Drawing for the job (mm, zero at the part's lowest x, y, z). Give positions to 0.01 mm unless a question says otherwise; leave off trailing zeros. Loops run counter-clockwise (first coordinate to the right, second up) from the corner with the lowest first, then second, coordinate; pieces in that order, holes last.
1) Band-saw the part on C-C on y = 2.45. List the corners of the cut face in (x, z).
2) Two-plate mould, pull along X, no slides. Class the marked faces 1, 2 and 3: +X half, -X half, draft (parallel to the pull), parting line (faces both ways), or undercut.
3) Band-saw the part on B-B on z = 28. List the corners of the cut face in (x, y).
4) Band-saw the part on A-A on x = 28. List the corners of the cut face in (y, z), then the cut area to 3 significant figures.
5) Wall check: line 1 (X direction, y = 3.95, z = 28); line 2 (X direction, y = 1.55, z = 34); line 3 (Z direction, x = 38.5, y = 4.9). Give the ranges that are in metal, low to high.
6) Flat gauge pin, fed straight in: P1, Ø3, axis at y = 4.5, z = 42, coming from the +X side. Where does the tip first touch, or does it go through?
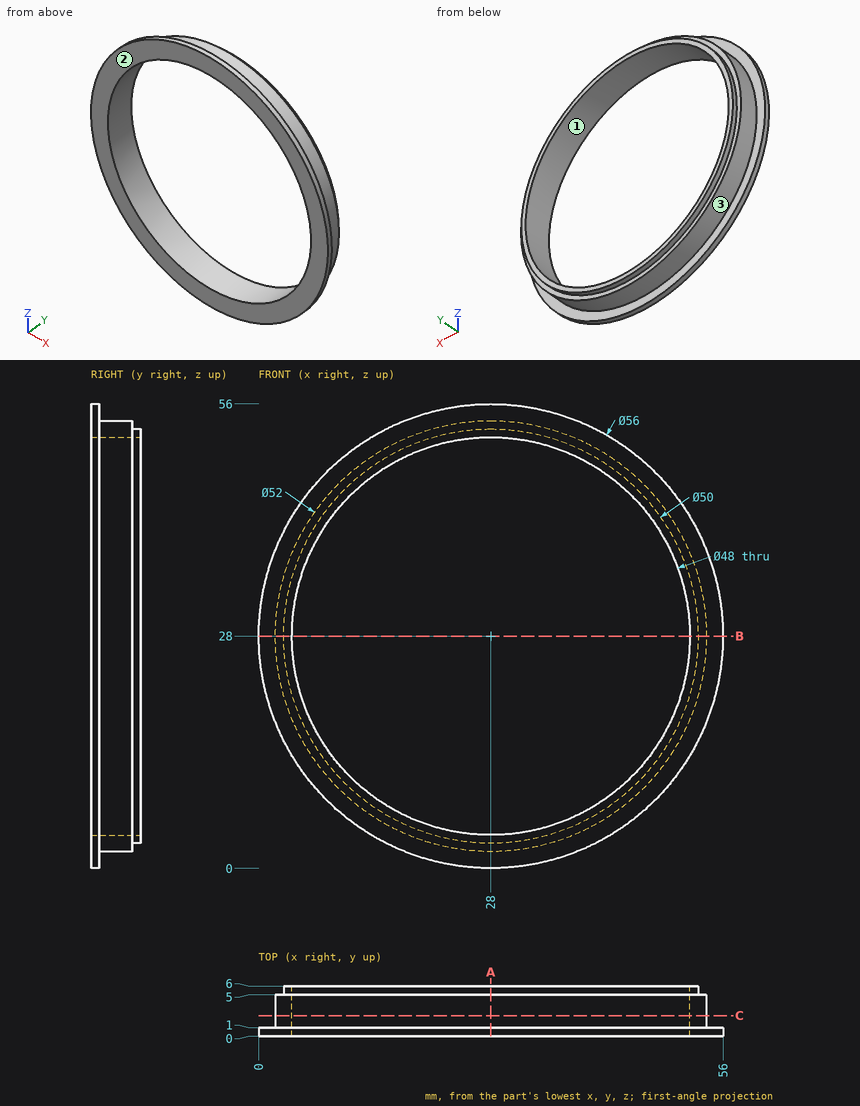
Findings below:
1. outline: circle Ø52 at (28, 28); hole circle Ø48 at (28, 28)
2. face 1: undercut
2. face 2: draft
2. face 3: parting line
3. outline: (0, 0) - (4, 0) - (4, 6) - (3, 6) - (3, 5) - (2, 5) - (2, 1) - (0, 1) - close; (52, 0) - (56, 0) - (56, 1) - (54, 1) - (54, 5) - (53, 5) - (53, 6) - (52, 6) - close
4. outline: (0, 0) - (1, 0) - (1, 2) - (5, 2) - (5, 3) - (6, 3) - (6, 4) - (0, 4) - close; (0, 52) - (6, 52) - (6, 53) - (5, 53) - (5, 54) - (1, 54) - (1, 56) - (0, 56) - close
4. area: 26.0 mm2
5. line 1: x = 2 to 4, 52 to 54
5. line 2: x = 2.7 to 4.76, 51.24 to 53.3
5. line 3: z = 4.21 to 6.42, 49.58 to 51.79
6. P1: stops at x = 50.8
